```python
from build123d import *

# Parameters (mm, degrees)
BOSS_EXTRUDE1_DEPTH            = 6.35
M5_CLEARANCE_HOLE1_D           = 5.5
M5_CLEARANCE_HOLE1_CSINK_D     = 5.55
M5_CLEARANCE_HOLE1_CSINK_ANGLE = 90
SKETCH5_R                      = 12.75
CUT_EXTRUDE1_DEPTH             = 53.941689622
CBORE_FOR_M4_SHCS1_AT_2_COUNT  = 2
CBORE_FOR_M4_SHCS1_AT_2_PITCH  = 21.169571299
FILLET1_R                      = 2


with BuildPart() as part:
    # Sketch1 → Boss-Extrude1 (new body)
    with BuildSketch(Plane(origin=(0, 0, 0), x_dir=(1, 0, 0), z_dir=(0, 1, 0))):
        with BuildLine():
            Line((-22.5, -47.5), (22.5, -47.5))
            Line((22.5, -47.5), (22.5, 3.34e-07))
            ThreePointArc((22.5, 3.34e-07), (0, 22.5), (-22.5, 3.34e-07))
            Line((-22.5, 3.34e-07), (-22.5, -47.5))
        make_face()
    extrude(amount=BOSS_EXTRUDE1_DEPTH)

    # M5 Clearance Hole1 (through all)
    with Locations(Plane(origin=(0, 6.35, 0), x_dir=(1, 0, 0), z_dir=(0, 1, 0))):
        with Locations((-6.696960066, -16.167891819), (6.696960066, -16.167891819), (6.696960066, 16.167891819), (-6.696960066, 16.167891819)):
            CounterSinkHole(M5_CLEARANCE_HOLE1_D / 2, M5_CLEARANCE_HOLE1_CSINK_D / 2, counter_sink_angle=M5_CLEARANCE_HOLE1_CSINK_ANGLE)

    # Sketch5 → Cut-Extrude1 (cut, through all)
    with BuildSketch(Plane(origin=(0, 6.35, 0), x_dir=(1, 0, 0), z_dir=(0, 1, 0))):
        with Locations(Location((0, 0, 0), (0, 0, 270))):
            Circle(SKETCH5_R)
    extrude(amount=-CUT_EXTRUDE1_DEPTH, mode=Mode.SUBTRACT)

    # Sketch10 → CBORE for M4 SHCS1 (revolve, cut)
    with BuildSketch(Plane(origin=(10.584785649, 0, 40.5), x_dir=(0, 0, -1), z_dir=(1, 0, 0))):
        Polygon((0, 0), (0, 6.35), (2.4, 6.35), (2.4, 4), (4, 4), (4, 0.025), (4.025, 0), align=None)
    cbore_for_m4_shcs1 = revolve(axis=Axis((10.584785649, -6.35, 40.5), (0, 1, 0)), mode=Mode.SUBTRACT)

    # CBORE for M4 SHCS1 at 2: CBORE for M4 SHCS1 ×2
    with Locations(*[(-i * CBORE_FOR_M4_SHCS1_AT_2_PITCH, 0, 0) for i in range(1, CBORE_FOR_M4_SHCS1_AT_2_COUNT)]):
        add(cbore_for_m4_shcs1, mode=Mode.SUBTRACT)

    # Fillet1
    fillet1_edges = [part.edges().sort_by_distance(p)[0] for p in [
        (22.5, 3.175, 47.5),
        (-22.5, 3.175, 47.5),
    ]]
    fillet(fillet1_edges, radius=FILLET1_R)


solid = part.part
```
Part model, mm, in its own coordinate system. A direction names the side the tool comes from. Round coordinates to 2 decimals unless told otherwise and drop trailing zeros. Loops run counter-clockwise (first coordinate to the right, second up) from the corner with the lowest first, then second, coordinate; pieces in that order, holes last. Notation, with made-up numbers: (-3, -21.75) -> (26, -21.75) arc R22 ccw to (26, 4.25) -> close; hole circle Ø6 at (14.5, 76.5). An arc over 180 degrees is marked (long way). Use a Markdown table: item, result.
1) Probe line 1 (X direction, y = 5.35, z = 40.5); line 2 (Z direction, x = -5.5, y = 3.5); line 3 (Z direction, x = 0.5, y = 5.5). List the from-to ranges inside material, lowest first. Write a range as [from, to].
The answers:
| item | result |
|---|---|
| line 1 | x = [-22.5, -12.98], [-8.18, 8.18], [12.98, 22.5] |
| line 2 | z = [-21.82, -18.64], [-13.69, -11.5], [11.5, 13.69], [18.64, 47.5] |
| line 3 | z = [-22.49, -12.74], [12.74, 47.5] |
2) Drop a flat-ended pin along its axis: pin 1 Ø6 at (x, z) = (10.58, 40.5) entering from -Y. Give the stop position or say it passes through.
The answers:
| item | result |
|---|---|
| pin 1 | stops at y = 4 |
3) Cut at D-D, the plane y = 1.75. List the corners of the cut face in (x, z), and give its area (3 significant figures).
The answers:
| item | result |
|---|---|
| outline | (-22.5, 0) arc R22.5 ccw to (22.5, 0) -> (22.5, 45.5) arc R2 ccw to (20.5, 47.5) -> (-20.5, 47.5) arc R2 ccw to (-22.5, 45.5) -> close; hole circle Ø8 at (-10.58, 40.5); hole circle Ø25.5 at (0, 0); hole circle Ø5.5 at (-6.7, -16.17); hole circle Ø5.5 at (-6.7, 16.17); hole circle Ø5.5 at (6.7, -16.17); hole circle Ø5.5 at (6.7, 16.17); hole circle Ø8 at (10.58, 40.5) |
| area | 2,220 mm2 |
4) Cut at A-A, the plane x = 0. List the corners of the cut face in (y, z), and give its area (3 significant figures).
The answers:
| item | result |
|---|---|
| outline | (0, -22.5) -> (6.35, -22.5) -> (6.35, -12.75) -> (0, -12.75) -> close; (0, 12.75) -> (6.35, 12.75) -> (6.35, 47.5) -> (0, 47.5) -> close |
| area | 283 mm2 |
5) Cut at C-C, the plane z = 8.5. List the corners of the cut face in (x, y).
The answers:
| item | result |
|---|---|
| outline | (-22.5, 0) -> (-9.5, 0) -> (-9.5, 6.35) -> (-22.5, 6.35) -> close; (9.5, 0) -> (22.5, 0) -> (22.5, 6.35) -> (9.5, 6.35) -> close |
6) Cut at B-B, the plane z = 40.5. List the corners of the cut face in (x, y) (3 decimals), and give its area (3 significant figures).
The answers:
| item | result |
|---|---|
| outline | (-22.5, 0) -> (-14.61, 0) -> (-14.585, 0.025) -> (-14.585, 4) -> (-12.985, 4) -> (-12.985, 6.35) -> (-22.5, 6.35) -> close; (-8.185, 4) -> (-6.585, 4) -> (-6.585, 0.025) -> (-6.56, 0) -> (6.56, 0) -> (6.585, 0.025) -> (6.585, 4) -> (8.185, 4) -> (8.185, 6.35) -> (-8.185, 6.35) -> close; (12.985, 4) -> (14.585, 4) -> (14.585, 0.025) -> (14.61, 0) -> (22.5, 0) -> (22.5, 6.35) -> (12.985, 6.35) -> close |
| area | 199 mm2 |
7) Pull direction X, two halves, no side cores. Call faces 1 (the flat face through (-10.6, 4, 43.1)), 2 (the flat face through (22.5, 3, 23)), 3 (the flat face through (0, 3, 47.5)): pulls with the +X half, pulls with the -X half, needs draft (parallel to the pull), parting line crosses it, or undercut.
The answers:
| item | result |
|---|---|
| face 1 | undercut |
| face 2 | pulls with the +X half |
| face 3 | needs draft |
8) Tool access for faces 4 (the flat face through (0, 6.35, 20)), 5 (the cylindrical face through (13.019, 1.985, 43.674)): list every direction of +Z, -Z, +X, -X, +Y, -Y with a clear straight run to the whole face (end or side of a thin tool).
The answers:
| item | result |
|---|---|
| face 4 | +Z, -Z, +X, -X, +Y |
| face 5 | -Y |
